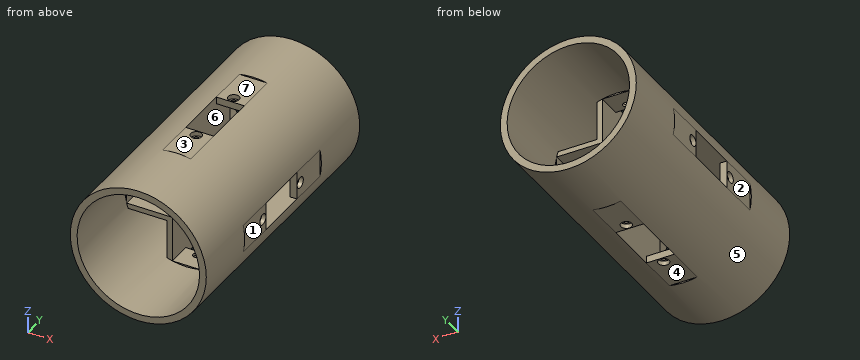
```python
from build123d import *

# Parameters (mm, degrees)
SKETCH_1_R               = 20
SKETCH_1_R_2             = 18
EXTRUDE_1_DEPTH          = 80
EXTRUDE_START            = 25
EXTRUDE_2_DEPTH          = 30
CUT_EXTRUDE_START        = 20
CUT_EXTRUDE_1_DEPTH      = 40
CUT_EXTRUDE_3_DEPTH      = 30
CUT_EXTRUDE_3_DEPTH_BACK = 30
SKETCH_4_W               = 8.2
SKETCH_4_H               = 16
SKETCH_4_R               = 1
CUT_EXTRUDE_4_DEPTH      = 30
CUT_EXTRUDE_4_DEPTH_BACK = 30
SKETCH_5_R               = 1
SKETCH_5_W               = 8.2
SKETCH_5_H               = 16
EXTRUDE_3_DEPTH          = 30
EXTRUDE_START_2          = 39
EXTRUDE_4_DEPTH          = 2
CUT_EXTRUDE_START_2      = 18.275239
SKETCH_8_R               = 1.6
CUT_EXTRUDE_5_DEPTH      = 1.300001
CUT_EXTRUDE_START_3      = -19.57524
SKETCH_9_R               = 1.6
CUT_EXTRUDE_6_DEPTH      = 1.300001
SKETCH_10_R              = 1.6
CUT_EXTRUDE_7_DEPTH      = 1.300001
SKETCH_11_R              = 1.6
CUT_EXTRUDE_8_DEPTH      = 1.300001


with BuildPart() as part:
    # 草图1 → 凸台-拉伸1 (new body)
    with BuildSketch(Plane(origin=(0, 0, 0), x_dir=(1, 0, 0), z_dir=(0, 1, 0))):
        with Locations(Location((0, 0, 0), (0, 0, 270))):
            Circle(SKETCH_1_R)
        with Locations(Location((0, 0, 0), (0, 0, 270))):
            Circle(SKETCH_1_R_2, mode=Mode.SUBTRACT)
    extrude(amount=EXTRUDE_1_DEPTH)

    # 草图2 → 凸台-拉伸2 (add)
    with BuildSketch(Plane(origin=(0, 0, 0), x_dir=(1, 0, 0), z_dir=(0, 1, 0)).offset(EXTRUDE_START)):
        with BuildLine():
            Line((17.526836566, 4.1), (17.526836566, -4.1))
            ThreePointArc((17.526836566, -4.1), (18, 0), (17.526836566, 4.1))
        make_face()
        with BuildLine():
            ThreePointArc((-4.1, -17.526836566), (0, -18), (4.1, -17.526836566))
            Line((4.1, -17.526836566), (-4.1, -17.526836566))
        make_face()
        with BuildLine():
            Line((-4.1, 17.526836566), (4.1, 17.526836566))
            ThreePointArc((4.1, 17.526836566), (0, 18), (-4.1, 17.526836566))
        make_face()
        with BuildLine():
            ThreePointArc((-17.526836566, 4.1), (-18, 0), (-17.526836566, -4.1))
            Line((-17.526836566, -4.1), (-17.526836566, 4.1))
        make_face()
    extrude(amount=EXTRUDE_2_DEPTH)

    # 草图3 → 切除-拉伸1 (cut)
    with BuildSketch(Plane(origin=(0, 0, 0), x_dir=(1, 0, 0), z_dir=(0, 1, 0)).offset(CUT_EXTRUDE_START)):
        with BuildLine():
            Line((-19.575239462, -4.1), (-19.575239462, 4.1))
            ThreePointArc((-19.575239462, 4.1), (-20, 0), (-19.575239462, -4.1))
        make_face()
        with BuildLine():
            Line((4.1, -19.575239462), (-4.1, -19.575239462))
            ThreePointArc((-4.1, -19.575239462), (0, -20), (4.1, -19.575239462))
        make_face()
        with BuildLine():
            ThreePointArc((20, 0), (19.89352645, 2.06097195), (19.575239462, 4.1))
            Line((19.575239462, 4.1), (19.575239462, -4.1))
            ThreePointArc((19.575239462, -4.1), (19.89352645, -2.06097195), (20, 0))
        make_face()
        with BuildLine():
            ThreePointArc((4.1, 19.575239462), (0, 20), (-4.1, 19.575239462))
            Line((-4.1, 19.575239462), (4.1, 19.575239462))
        make_face()
    extrude(amount=CUT_EXTRUDE_1_DEPTH, mode=Mode.SUBTRACT)

    # 草图4 → 切除-拉伸3 (cut, two sides: drawn at the far end of the back side and taken through both)
    with BuildSketch(Plane.XY.offset(-CUT_EXTRUDE_3_DEPTH_BACK)):
        with Locations((0, 40)):
            Rectangle(SKETCH_4_W, SKETCH_4_H)
        with Locations(Location((0, 49.75, 0), (0, 0, 180))):
            Circle(SKETCH_4_R)
        with Locations(Location((0, 30.25, 0), (0, 0, 180))):
            Circle(SKETCH_4_R)
    extrude(amount=CUT_EXTRUDE_3_DEPTH + CUT_EXTRUDE_3_DEPTH_BACK, mode=Mode.SUBTRACT)

    # 草图5 → 切除-拉伸4 (cut, two sides: drawn at the far end of the back side and taken through both)
    with BuildSketch(Plane(origin=(0, 0, 0), x_dir=(0, 0, -1), z_dir=(1, 0, 0)).offset(-CUT_EXTRUDE_4_DEPTH_BACK)):
        with Locations((0, 49.75)):
            Circle(SKETCH_5_R)
        with Locations((0, 30.25)):
            Circle(SKETCH_5_R)
        with Locations((0, 40)):
            Rectangle(SKETCH_5_W, SKETCH_5_H)
    extrude(amount=CUT_EXTRUDE_4_DEPTH + CUT_EXTRUDE_4_DEPTH_BACK, mode=Mode.SUBTRACT)

    # 草图6 → 凸台-拉伸3 (add)
    with BuildSketch(Plane(origin=(0, 0, 0), x_dir=(1, 0, 0), z_dir=(0, 1, 0)).offset(EXTRUDE_START)):
        with BuildLine():
            Line((-4.1, 4.1), (-4.1, 17.526836566))
            ThreePointArc((-4.1, 17.526836566), (-4.854546702, 17.333014058), (-5.6, 17.106723824))
            Line((-5.6, 17.106723824), (-5.6, 5.6))
            Line((-5.6, 5.6), (-17.106723824, 5.6))
            ThreePointArc((-17.106723824, 5.6), (-17.333014058, 4.854546702), (-17.526836566, 4.1))
            Line((-17.526836566, 4.1), (-4.1, 4.1))
        make_face()
        with BuildLine():
            Line((4.1, 4.1), (17.526836566, 4.1))
            ThreePointArc((17.526836566, 4.1), (17.333014058, 4.854546702), (17.106723824, 5.6))
            Line((17.106723824, 5.6), (5.6, 5.6))
            Line((5.6, 5.6), (5.6, 17.106723824))
            ThreePointArc((5.6, 17.106723824), (4.854546702, 17.333014058), (4.1, 17.526836566))
            Line((4.1, 17.526836566), (4.1, 4.1))
        make_face()
        with BuildLine():
            ThreePointArc((17.106723824, -5.6), (17.333014058, -4.854546702), (17.526836566, -4.1))
            Line((17.526836566, -4.1), (4.1, -4.1))
            Line((4.1, -4.1), (4.1, -17.526836566))
            ThreePointArc((4.1, -17.526836566), (4.854546702, -17.333014058), (5.6, -17.106723824))
            Line((5.6, -17.106723824), (5.6, -5.6))
            Line((5.6, -5.6), (17.106723824, -5.6))
        make_face()
        with BuildLine():
            ThreePointArc((-5.6, -17.106723824), (-4.854546702, -17.333014058), (-4.1, -17.526836566))
            Line((-4.1, -17.526836566), (-4.1, -4.1))
            Line((-4.1, -4.1), (-17.526836566, -4.1))
            ThreePointArc((-17.526836566, -4.1), (-17.333014058, -4.854546702), (-17.106723824, -5.6))
            Line((-17.106723824, -5.6), (-5.6, -5.6))
            Line((-5.6, -5.6), (-5.6, -17.106723824))
        make_face()
    extrude(amount=EXTRUDE_3_DEPTH)

    # 草图7 → 凸台-拉伸4 (add)
    # profile 1 of 5: a face of its own
    with BuildSketch(Plane(origin=(0, 0, 0), x_dir=(1, 0, 0), z_dir=(0, 1, 0)).offset(EXTRUDE_START_2)):
        with BuildLine():
            Line((5.6, 5.6), (17.106723824, 5.6))
            ThreePointArc((17.106723824, 5.6), (12.727922061, 12.727922061), (5.6, 17.106723824))
            Line((5.6, 17.106723824), (5.6, 5.6))
        make_face()
        with BuildLine():
            Line((6.865863992, 8.280077554), (10.047844507, 11.46205807))
            ThreePointArc((10.047844507, 11.46205807), (11.46205807, 11.46205807), (11.46205807, 10.047844507))
            Line((11.46205807, 10.047844507), (8.280077554, 6.865863992))
            ThreePointArc((8.280077554, 6.865863992), (6.865863992, 6.865863992), (6.865863992, 8.280077554))
        make_face(mode=Mode.SUBTRACT)
    # profile 2 of 5: a face of its own
    with BuildSketch(Plane(origin=(0, 0, 0), x_dir=(1, 0, 0), z_dir=(0, 1, 0)).offset(EXTRUDE_START_2)):
        with BuildLine():
            Line((17.106723824, -5.6), (5.6, -5.6))
            Line((5.6, -5.6), (5.6, -17.106723824))
            ThreePointArc((5.6, -17.106723824), (12.727922061, -12.727922061), (17.106723824, -5.6))
        make_face()
        with BuildLine():
            ThreePointArc((11.46205807, -10.047844507), (11.46205807, -11.46205807), (10.047844507, -11.46205807))
            Line((10.047844507, -11.46205807), (6.865863992, -8.280077554))
            ThreePointArc((6.865863992, -8.280077554), (6.865863992, -6.865863992), (8.280077554, -6.865863992))
            Line((8.280077554, -6.865863992), (11.46205807, -10.047844507))
        make_face(mode=Mode.SUBTRACT)
    # profile 3 of 5: a face of its own
    with BuildSketch(Plane(origin=(0, 0, 0), x_dir=(1, 0, 0), z_dir=(0, 1, 0)).offset(EXTRUDE_START_2)):
        with BuildLine():
            ThreePointArc((-17.106723824, -5.6), (-12.727922061, -12.727922061), (-5.6, -17.106723824))
            Line((-5.6, -17.106723824), (-5.6, -5.6))
            Line((-5.6, -5.6), (-17.106723824, -5.6))
        make_face()
        with BuildLine():
            Line((-6.865863992, -8.280077554), (-10.047844507, -11.46205807))
            ThreePointArc((-10.047844507, -11.46205807), (-11.46205807, -11.46205807), (-11.46205807, -10.047844507))
            Line((-11.46205807, -10.047844507), (-8.280077554, -6.865863992))
            ThreePointArc((-8.280077554, -6.865863992), (-6.865863992, -6.865863992), (-6.865863992, -8.280077554))
        make_face(mode=Mode.SUBTRACT)
    # profile 4 of 5: a face of its own
    with BuildSketch(Plane(origin=(0, 0, 0), x_dir=(1, 0, 0), z_dir=(0, 1, 0)).offset(EXTRUDE_START_2)):
        with BuildLine():
            Line((-5.6, 5.6), (-5.6, 17.106723824))
            ThreePointArc((-5.6, 17.106723824), (-9.421871257, 15.337155604), (-12.727922061, 12.727922061))
            Line((-12.727922061, 12.727922061), (-11.46205807, 11.46205807))
            ThreePointArc((-11.46205807, 11.46205807), (-10.754951288, 11.754951288), (-10.047844507, 11.46205807))
            Line((-10.047844507, 11.46205807), (-6.865863992, 8.280077554))
            ThreePointArc((-6.865863992, 8.280077554), (-6.572970773, 7.572970773), (-6.865863992, 6.865863992))
            Line((-6.865863992, 6.865863992), (-5.6, 5.6))
        make_face()
    # profile 5 of 5: a face of its own
    with BuildSketch(Plane(origin=(0, 0, 0), x_dir=(1, 0, 0), z_dir=(0, 1, 0)).offset(EXTRUDE_START_2)):
        with BuildLine():
            ThreePointArc((-12.727922061, 12.727922061), (-15.337155604, 9.421871257), (-17.106723824, 5.6))
            Line((-17.106723824, 5.6), (-5.6, 5.6))
            Line((-5.6, 5.6), (-6.865863992, 6.865863992))
            ThreePointArc((-6.865863992, 6.865863992), (-7.572970773, 6.572970773), (-8.280077554, 6.865863992))
            Line((-8.280077554, 6.865863992), (-11.46205807, 10.047844507))
            ThreePointArc((-11.46205807, 10.047844507), (-11.754951288, 10.754951288), (-11.46205807, 11.46205807))
            Line((-11.46205807, 11.46205807), (-12.727922061, 12.727922061))
        make_face()
    extrude(amount=EXTRUDE_4_DEPTH)

    # 草图8 → 切除-拉伸5 (cut)
    with BuildSketch(Plane.XY.offset(CUT_EXTRUDE_START_2)):
        with Locations(Location((0, 49.75, 0), (0, 0, 180))):
            Circle(SKETCH_8_R)
        with Locations(Location((0, 30.25, 0), (0, 0, 180))):
            Circle(SKETCH_8_R)
    extrude(amount=CUT_EXTRUDE_5_DEPTH, mode=Mode.SUBTRACT)

    # 草图9 → 切除-拉伸6 (cut)
    with BuildSketch(Plane.XY.offset(CUT_EXTRUDE_START_3)):
        with Locations(Location((0, 49.75, 0), (0, 0, 180))):
            Circle(SKETCH_9_R)
        with Locations(Location((0, 30.25, 0), (0, 0, 180))):
            Circle(SKETCH_9_R)
    extrude(amount=CUT_EXTRUDE_6_DEPTH, mode=Mode.SUBTRACT)

    # 草图10 → 切除-拉伸7 (cut)
    with BuildSketch(Plane(origin=(0, 0, 0), x_dir=(0, 0, -1), z_dir=(1, 0, 0)).offset(CUT_EXTRUDE_START_3)):
        with Locations((0, 49.75)):
            Circle(SKETCH_10_R)
        with Locations((0, 30.25)):
            Circle(SKETCH_10_R)
    extrude(amount=CUT_EXTRUDE_7_DEPTH, mode=Mode.SUBTRACT)

    # 草图11 → 切除-拉伸8 (cut)
    with BuildSketch(Plane(origin=(0, 0, 0), x_dir=(0, 0, -1), z_dir=(1, 0, 0)).offset(CUT_EXTRUDE_START_2)):
        with Locations((0, 49.75)):
            Circle(SKETCH_11_R)
        with Locations((0, 30.25)):
            Circle(SKETCH_11_R)
    extrude(amount=CUT_EXTRUDE_8_DEPTH, mode=Mode.SUBTRACT)


solid = part.part
```
Design review of the part built by this model. Coordinates are the model's own, in mm. Face numbers are marked on the shaded views. A direction names the side the tool comes from. Give positions to 0.01 mm unless a question says otherwise; leave off trailing zeros. Write each loop counter-clockwise with the first axis right and the second up, starting at its lowest first coordinate (ties: lowest second). Pieces come first, ordered by that corner, then holes. Notation, with made-up numbers: (0, 49) -> (6, 49) arc R28 ccw to (6, 80) -> close; hole circle Ø1 at (-32, 17.5). An arc over 180 degrees is marked (long way). Answer in a Markdown table with one row per item.
(1) Mouldability with a two-part tool opening along X and no side actions: class the marked faces 5, 6 and 7 as +X half, -X half, draft (parallel to the pull), parting line (faces both ways), or undercut.
Results:
| item | result |
|---|---|
| face 5 | parting line |
| face 6 | undercut |
| face 7 | draft |
(2) Clearance check with flat-ended pins moving along their axes: pin 1 (6.5 mm diameter, centred on y = 56, z = -0.5, fed in from +X); pin 2 (4 mm diameter, centred on x = -14, y = 51, fed in from +Z); pin 3 (12.5 mm diameter, centred on x = 11, y = 47.5, fed in from -Z). State where each tip first meets the part, or that it passes through.
Results:
| item | result |
|---|---|
| pin 1 | x = 19.58 |
| pin 2 | z = 16 |
| pin 3 | z = -19.43 |
(3) Consider section A-A (y = 34.5). State the section outline as (x, z) points.
Results:
| item | result |
|---|---|
| outline | (-19.58, -4.1) arc R20 ccw to (-4.1, -19.58) -> (-4.1, -4.1) -> close; (-19.58, 4.1) -> (-4.1, 4.1) -> (-4.1, 19.58) arc R20 ccw to start; (4.1, -19.58) arc R20 ccw to (19.58, -4.1) -> (4.1, -4.1) -> close; (4.1, 4.1) -> (19.58, 4.1) arc R20 ccw to (4.1, 19.58) -> close; hole (-17.11, -5.6) arc R18 ccw to (-5.6, -17.11) -> (-5.6, -5.6) -> close; hole (-17.11, 5.6) -> (-5.6, 5.6) -> (-5.6, 17.11) arc R18 ccw to start; hole (5.6, -17.11) arc R18 ccw to (17.11, -5.6) -> (5.6, -5.6) -> close; hole (5.6, 5.6) -> (17.11, 5.6) arc R18 ccw to (5.6, 17.11) -> close |
(4) Consider section D-D (z = -16). State the section outline as (x, y) points.
Results:
| item | result |
|---|---|
| outline | (-12, 0) -> (-8.25, 0) -> (-8.25, 39) -> (-5.6, 39) -> (-5.6, 25) -> (-4.1, 25) -> (-4.1, 55) -> (-5.6, 55) -> (-5.6, 41) -> (-8.25, 41) -> (-8.25, 80) -> (-12, 80) -> close; (4.1, 25) -> (5.6, 25) -> (5.6, 39) -> (8.25, 39) -> (8.25, 0) -> (12, 0) -> (12, 80) -> (8.25, 80) -> (8.25, 41) -> (5.6, 41) -> (5.6, 55) -> (4.1, 55) -> close |
(5) To check wall thickness, follow probe 1 along Y at (x, z) = (18.7, 0); probe 2 along X at (y, z) = (40, 9); probe 3 along X at (y, z) = (32.5, 11). State the ranges of each line that lie inside material, in increasing order.
Results:
| item | result |
|---|---|
| probe 1 | 0 to 28.65, 31.85 to 32, 48 to 48.15, 51.35 to 80 |
| probe 2 | -17.86 to -10.41, -7.59 to -4.1, 4.1 to 7.59, 10.41 to 17.86 |
| probe 3 | -16.7 to -14.25, -5.6 to -4.1, 4.1 to 5.6, 14.25 to 16.7 |
(6) For the marked faces 1, 2, 3 and 4, list the 3-axis set-ups (+Z, -Z, +X, -X, +Y, -Y) from which the entire face can be reached by the end or side of a thin tool; tool diameter is ignored.
Results:
| item | result |
|---|---|
| face 1 | +Z, -Z, +X |
| face 2 | +Z, -Z, -X |
| face 3 | +Z, +X, -X |
| face 4 | -Z, +X, -X |
(7) Consider section B-B (z = 0). Count the separate pieces of the cut face and the enclosed holes in it, then the cut area to 3 significant figures.
Results:
| item | result |
|---|---|
| separate pieces | 8 |
| enclosed holes | 0 |
| area | 226 mm2 |
